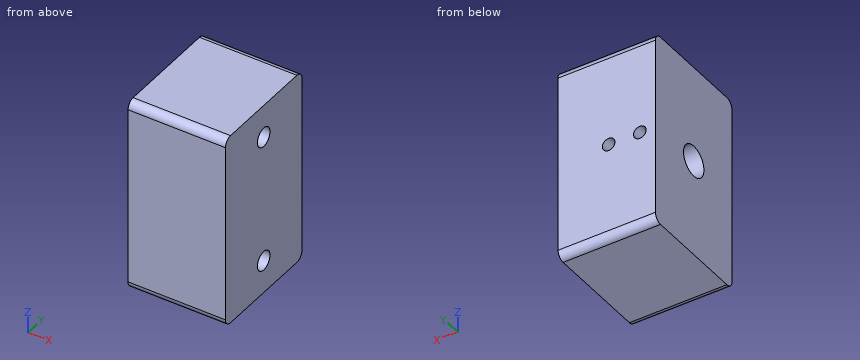
Autodesk Inventor part; units mm, degrees
ref_plane "YZ Plane" through (0, 0, 0) normal (1, 0, 0) x (0, 1, 0)
ref_plane "XZ Plane" through (0, 0, 0) normal (0, 1, 0) x (-1, 0, 0)
ref_plane "XY Plane" through (0, 0, 0) normal (0, 0, 1) x (1, 0, 0)
sketch "Sketch1" plane through (0, 0, 0) normal (1, 0, 0) x (0, 1, 0)
  line L0 (-15, 25) -> (15, 25)
  line L1 (15, 25) -> (15, -25)
  line L2 (15, -25) -> (-15, -25)
  line L3 (-15, -25) -> (-15, 25)
  line L4 (-15, 25) -> (15, -25) construction
  line L5 (15, 25) -> (-15, -25) construction
  point P0 (0, 0)
  dimension "d1" = 50
  dimension "d2" = 30
extrude "Extrusion1" add sketch "Sketch1" along normal blind 25
hole "Hole1" at (0, 0, 0) direction (1, 0, 0) diameter 8 depth 20
sketch "Sketch2" plane through (0, 15, 25) normal (0, 1, 0) x (1, 0, 0)
  line L0 (0, 25) -> (25, 25) construction
  line L1 (25, 50) -> (25, 0) construction
  line L2 (0, 50) -> (0, 0) construction
  point P0 (4, 25)
  point P1 (12, 25)
  dimension "d12" = 4
  dimension "d13" = 12
hole "Hole2" at (4, 15, 0) at (12, 15, 0) direction (0, -1, 0) diameter 3.242 end up to surface
sketch "Sketch3" plane through (25, 0, 0) normal (1, 0, 0) x (0, 0, -1)
  line L0 (-16.5, 0) -> (0, 0) construction
  line L1 (0, 0) -> (16.5, 0) construction
  dimension "d21" = 33
hole "Hole3" at (25, 0, 16.5) at (25, 0, -16.5) direction (-1, 0, 0) diameter 4.917 depth 17.1 tip angle 118
fillet "Fillet1" radius 2 4 edges at (12.5, 15, -25) (12.5, -15, -25) (12.5, -15, 25) (12.5, 15, 25)
properties part number "axle_tube_mount_8mm" material "Steel, Alloy"
Geometry check sheet. Reference: the model listing, model coordinates, mm. Give positions to 0.01 mm unless a question says otherwise; leave off trailing zeros. Order: outer loops, then holes, each group sorted by start corner. A loop starts at its lowest first (then second) coordinate and runs counter-clockwise, first axis right, second up. Notation, with made-up numbers: (83.25, 39) - (131.25, 39) arc R18 ccw to (131.25, 63) - close; hole circle Ø3 at (80.25, -32). An arc over 180 degrees is marked (long way). Answer as a JSON object with one key per item and string values.
(1) Cross-section at C-C (x = 4). Record the cut outline in (y, z), then the cut area to 3 significant figures.
Report:
{"outline": "(-15, -23) arc R2 ccw to (-13, -25) - (13, -25) arc R2 ccw to (15, -23) - (15, -1.62) - (3.66, -1.62) arc R4 cw (long way) to (3.66, 1.62) - (15, 1.62) - (15, 23) arc R2 ccw to (13, 25) - (-13, 25) arc R2 ccw to (-15, 23) - close", "area": "1,410 mm^2"}
(2) Depth check by flat-ended pin: pin 1 Ø4 at (y, z) = (0, -16.5) entering from +X; pin 2 Ø4 at (y, z) = (-1, 0) entering from -X; pin 3 Ø1.9 at (x, z) = (12, 0) entering from +Y. Enter the tip coordinate at first touch or a pass-through.
Report:
{"pin 1": "x = 7.62", "pin 2": "x = 20", "pin 3": "y = -3.89"}
(3) Material ranges on line 1 (X direction, y = 8.5, z = 0); line 2 (Z direction, x = 19.25, y = 0); line 3 (Z direction, x = 4, y = 9.25), recorded low to high.
Report:
{"line 1": "0 to 2.38, 5.62 to 10.38, 13.62 to 25", "line 2": "-25 to -18.96, -14.04 to -4, 4 to 14.04, 18.96 to 25", "line 3": "-25 to -1.62, 1.62 to 25"}
(4) Cross-section at A-A (x = 16.75). Record the cut outline in (y, z), then the cut area to 3 significant figures.
Report:
{"outline": "(-15, -23) arc R2 ccw to (-13, -25) - (13, -25) arc R2 ccw to (15, -23) - (15, 23) arc R2 ccw to (13, 25) - (-13, 25) arc R2 ccw to (-15, 23) - close; hole circle Ø8 at (0, 0); hole circle Ø4.92 at (0, -16.5); hole circle Ø4.92 at (0, 16.5)", "area": "1,410 mm^2"}
(5) Cross-section at B-B (z = 0). Record the cut outline in (x, y).
Report:
{"outline": "(0, -15) - (25, -15) - (25, 15) - (13.62, 15) - (13.62, 4) - (20, 4) - (20, -4) - (0, -4) - close; (0, 4) - (2.38, 4) - (2.38, 15) - (0, 15) - close; (5.62, 4) - (10.38, 4) - (10.38, 15) - (5.62, 15) - close"}
